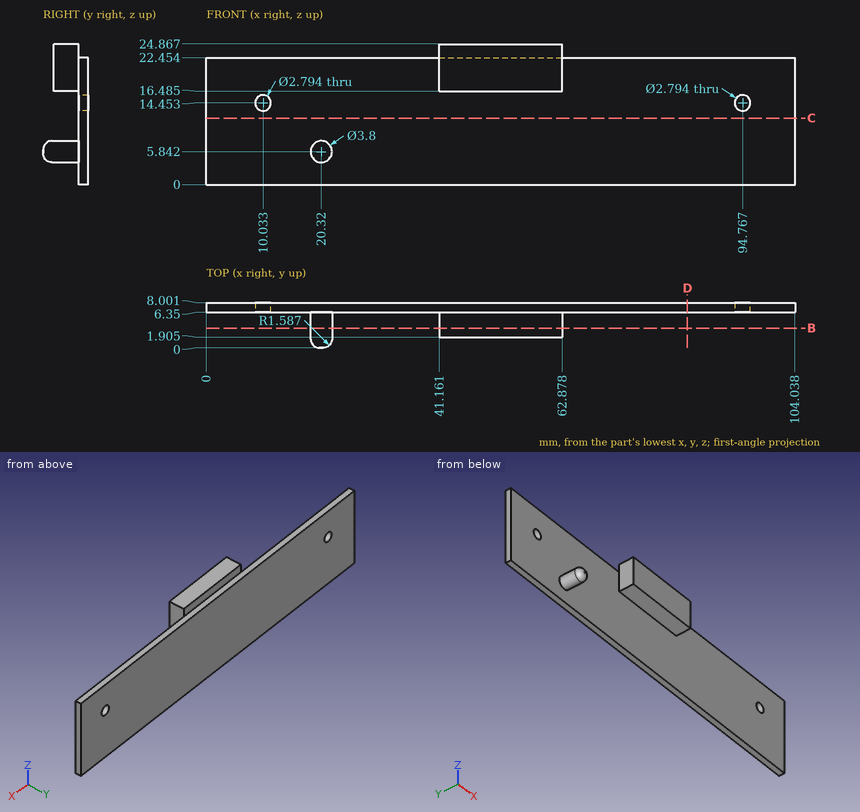
Study the drawing (mm; zero at the part's minimum x, y, z) and answer. Coordinates: 2 decimals unless noted, no trailing zeros. Loops run counter-clockwise (first coordinate to the right, second up) from the corner with the lowest first, then second, coordinate; pieces in that order, holes last. Notation, with made-up numbers: M 1,21 L 35,21 A26 ccw 35,42 Z; hole C 15,64 d10. An arc over 180 degrees is marked long. Answer in a Markdown table with one row per item. Add a question column.
1. Find section D-D, the plane x = 85. Write down the section's boundary in (y, z).
2. Flat-ended cylindrical pins translate along their axes: P1, Ø0.7, axis at x = 47, z = 23.5, coming from the +Y side; P2, Ø1.3, axis at x = 47, y = 4.5, coming from the -Z side (1 decimal); P3, Ø10, axis at x = 61, z = 6.5, coming from the -Y side. Find the tip coordinate at first contact, or state that the pin passes through.
3. Find section B-B, the plane y = 3.5. Write down the section's boundary in (x, z) (1 decimal).
4. Find section C-C, the plane z = 11.75. Write down the section's boundary in (x, y), then the cut area to 3 significant figures.
5. Consider L1, parallel to X at y = 4, z = 19; L2, parallel to Y at x = 60.5, z = 5; L3, parallel to Z at x = 51, y = 4 (1 decimal). Determine where each line is inside the solid, lowest interval first.
Reported:
| question | item | result |
|---|---|---|
| 1 | outline | M 6.35,0 L 8,0 L 8,22.45 L 6.35,22.45 Z |
| 2 | P1 | stops at y = 6.35 |
| 2 | P2 | stops at z = 16.5 |
| 2 | P3 | stops at y = 6.35 |
| 3 | outline | C 20.3,5.8 d3.8; M 41.2,16.5 L 62.9,16.5 L 62.9,24.9 L 41.2,24.9 Z |
| 4 | outline | M 0,6.35 L 104.04,6.35 L 104.04,8 L 0,8 Z |
| 4 | area | 172 mm^2 |
| 5 | L1 | x = 41.16 to 62.88 |
| 5 | L2 | y = 6.35 to 8 |
| 5 | L3 | z = 16.5 to 24.9 |
